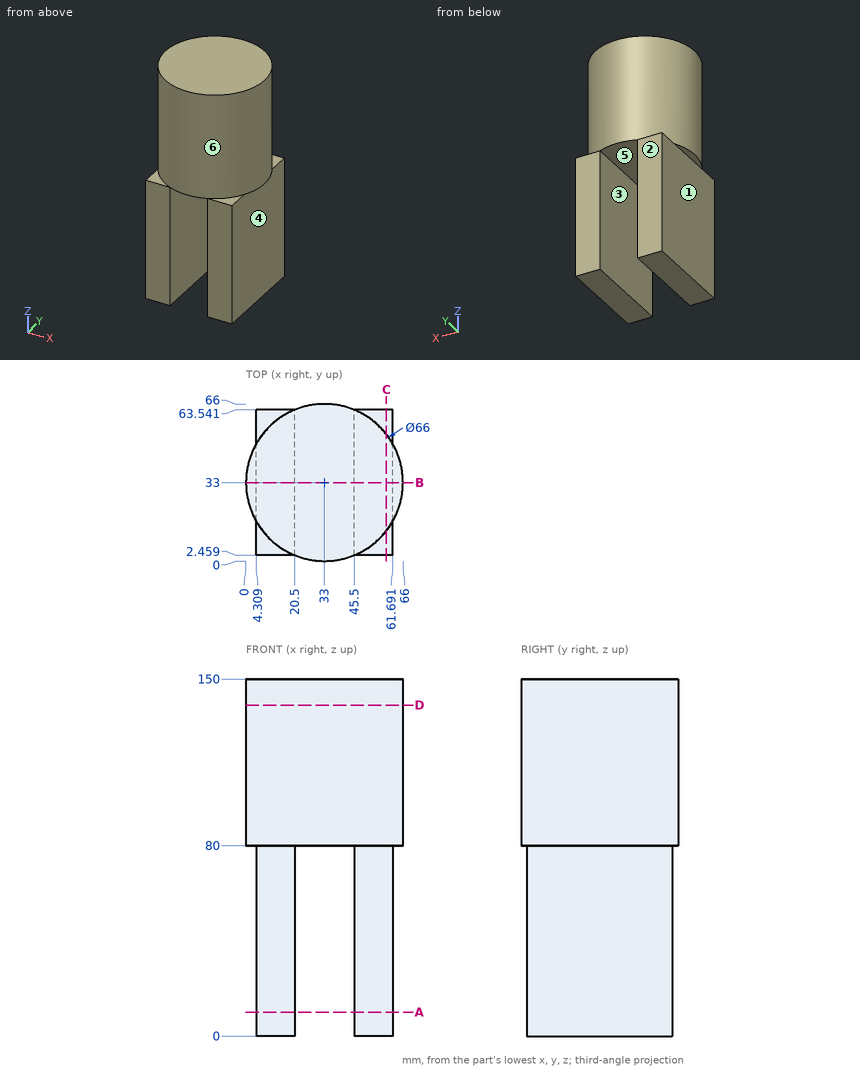
Source: three-view drawing plus pictorial views. Frame: mm from the lowest corner of the part. A direction names the side the tool comes from. Give positions to 0.01 mm unless a question says otherwise; leave off trailing zeros. Write each loop counter-clockwise with the first axis right and the second up, starting at its lowest first coordinate (ties: lowest second). Pieces come first, ordered by that corner, then holes. Notation, with made-up numbers: (28, 51) - (35, 51) arc R24 cw to (35, 88) - close; hole circle Ø9 at (77.5, -4.75). An arc over 180 degrees is marked (long way). Write item = value, one per line. Start each with the question number.
1. Section query D-D, the plane z = 139. Output: boundary loops of the cut face in (x, y).
2. Section query A-A, the plane z = 10. Output: boundary loops of the cut face in (x, y).
3. Section query C-C, the plane x = 59. Output: boundary loops of the cut face in (y, z).
4. Mould query, pull axis X, two halves, no side actions, for the marked faces 1, 2 and 3. Classes: released by +X, released by -X, zero draft, split by the parting line, or undercut.
5. First-contact query: pin 1 Ø2 at (x, z) = (48, 96) entering from +Y; pin 2 Ø4 at (x, y) = (29, 11) entering from -Z; pin 3 Ø10 at (x, z) = (48, 31.5) entering from -Y. Flat tips, straight axial feed; report the tip coordinate or a pass-through.
6. Ray query, L1, parallel to X at y = 24.5, z = 38; L2, parallel to Z at x = 42.5, y = 13; L3, parallel to Y at x = 20.5, z = 82. Return the intervals inside material, ascending.
7. Access query for the marked faces 4, 5 and 6. Directions: +Z, -Z, +X, -X, +Y, -Y. A direction counts if a zero-diameter tool reaches every point of the face in a straight line with its end or side. Return the directions, or none.
8. Section query B-B, the plane y = 33. Output: boundary loops of the cut face in (x, z).
Check sheet entries:
q1.outline = circle Ø66 at (33, 33)
q2.outline = (4.31, 2.46) - (20.5, 2.46) - (20.5, 63.54) - (4.31, 63.54) - close; (45.5, 2.46) - (61.69, 2.46) - (61.69, 63.54) - (45.5, 63.54) - close
q3.outline = (2.46, 0) - (63.54, 0) - (63.54, 80) - (53.32, 80) - (53.32, 150) - (12.68, 150) - (12.68, 80) - (2.46, 80) - close
q4.face_1 = released by -X
q4.face_2 = zero draft
q4.face_3 = undercut
q5.pin_1 = 62.88
q5.pin_2 = 80
q5.pin_3 = 2.46
q6.L1 = 4.31 to 20.5, 45.5 to 61.69
q6.L2 = 80 to 150
q6.L3 = 2.46 to 63.54
q7.face_4 = -Z, +X, +Y, -Y
q7.face_5 = -Z, +Y, -Y
q7.face_6 = +Z
q8.outline = (0, 80) - (4.31, 80) - (4.31, 0) - (20.5, 0) - (20.5, 80) - (45.5, 80) - (45.5, 0) - (61.69, 0) - (61.69, 80) - (66, 80) - (66, 150) - (0, 150) - close
